Autodesk Inventor part; units mm, degrees
ref_plane "YZ Plane" through (0, 0, 0) normal (1, 0, 0) x (0, 1, 0)
ref_plane "XZ Plane" through (0, 0, 0) normal (0, 1, 0) x (-1, 0, 0)
ref_plane "XY Plane" through (0, 0, 0) normal (0, 0, 1) x (1, 0, 0)
sketch "Sketch1" plane through (0, 0, 0) normal (0, 0, 1) x (1, 0, 0)
  spline S0 degree 3 poles (-30, -5) (-30, -4.3586) (-29.8694, -3.6802) (-29.3471, -2.4395) (-28.9555, -1.8763) (-28.0866, -1.0236) (-27.5672, -0.665) (-27, -0.4174) knots 1.621626 1.621626 1.621626 1.621626 1.814042 1.814042 2.006457 2.006457 2.182648 2.182648 2.182648 2.182648
  line L0 (-25, 0) -> (25, 0)
  spline S1 degree 3 poles (27, -0.4174) (27.5672, -0.665) (28.0866, -1.0236) (28.9555, -1.8763) (29.3471, -2.4395) (29.8694, -3.6802) (30, -4.3586) (30, -5) knots -0.561022 -0.561022 -0.561022 -0.561022 -0.384831 -0.384831 -0.192415 -0.192415 0 0 0 0
  line L1 (30, -5) -> (30, -35)
  spline S2 degree 3 poles (30, -35) (30, -35.6414) (29.8694, -36.3198) (29.3471, -37.5605) (28.9555, -38.1237) (28.0866, -38.9764) (27.5672, -39.335) (27, -39.5826) knots 0 0 0 0 0.192415 0.192415 0.384831 0.384831 0.561022 0.561022 0.561022 0.561022
  line L2 (25, -40) -> (-25, -40)
  line L3 (-30, -35) -> (-30, -5)
  spline S3 degree 3 poles (-27, -39.5826) (-27.5672, -39.335) (-28.0866, -38.9764) (-28.9555, -38.1237) (-29.3471, -37.5605) (-29.8694, -36.3198) (-30, -35.6414) (-30, -35) knots 1.060605 1.060605 1.060605 1.060605 1.236796 1.236796 1.429211 1.429211 1.621626 1.621626 1.621626 1.621626
  arc A0 (-25, 0) -> (-27, -0.4174) centre (-25, -5) ccw
  arc A1 (27, -0.4174) -> (25, 0) centre (25, -5) ccw
  arc A2 (25, -40) -> (27, -39.5826) centre (25, -35) ccw
  arc A3 (-27, -39.5826) -> (-25, -40) centre (-25, -35) ccw
  point P0 (0, 0)
  dimension "d8" = 60
  dimension "d9" = 40
extrude "Extrusion1" add sketch "Sketch1" along normal blind 0.8
sketch "Sketch2" plane through (0, 0, 0) normal (0, 0, -1) x (-1, 0, 0)
  line L0 (-25.5, -10) -> (25.5, -10)
  line L1 (25.5, -10) -> (25.5, -30)
  line L2 (25.5, -30) -> (-25.5, -30)
  line L3 (-25.5, -30) -> (-25.5, -10)
  line L4 (-25.5, -10) -> (25.5, -30) construction
  line L5 (25.5, -10) -> (-25.5, -30) construction
  line L6 (-26.5, -9) -> (26.5, -9)
  line L7 (26.5, -9) -> (26.5, -31)
  line L8 (26.5, -31) -> (-26.5, -31)
  line L9 (-26.5, -31) -> (-26.5, -9)
  line L10 (-26.5, -9) -> (26.5, -31) construction
  line L11 (26.5, -9) -> (-26.5, -31) construction
  point P0 (0, 0)
  point P1 (0, -20)
  point P2 (0, -20)
  dimension "d2" = 51
  dimension "d3" = 20
  dimension "d4" = 53
  dimension "d5" = 22
extrude "Extrusion2" add sketch "Sketch2" along normal blind 2
properties part number "obudowa - budzik v7 plexi" material "Glass"
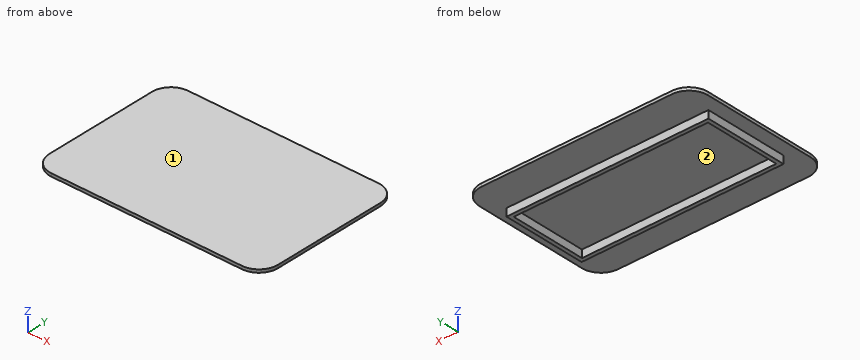
Verification items for the finished model (mm, model axes). Face numbers are marked on the shaded views. Give positions to 0.01 mm unless a question says otherwise; leave off trailing zeros. Order: outer loops, then holes, each group sorted by start corner. A loop starts at its lowest first (then second) coordinate and runs counter-clockwise, first axis right, second up. Notation, with made-up numbers: M -22,-15 L 27,-15 A16 ccw 27,-11 Z; hole C 33,-29.5 d9. An arc over 180 degrees is marked long. Answer as a JSON object with one key per item and string values. Group by question number.
1) Cross-section at A-A (x = -4). Enter the section's corners in (y, z), then the cut area to 3 significant figures.
2) Mould release check, pull along X, two halves, no side actions. Record for the marked faces 1 and 2: released by +X, released by -X, zero draft, split by the parting line, or undercut.
3) Depth check by flat-ended pin: pin 1 Ø1 at (x, z) = (-11, -1) entering from +Y; pin 2 Ø0.6 at (y, z) = (-25, -1) entering from -X; pin 3 Ø16 at (x, y) = (4.5, -21.5) entering from -Z. Enter the tip coordinate at first touch or a pass-through.
4) Cross-section at B-B (y = -20). Enter the section's corners in (x, z).
5) Cross-section at C-C (y = -32). Enter the section's corners in (x, z).
6) Scan lines: line 1 along Y through (x, z) = (-9, -1.2); line 2 along X through (y, z) = (-25, -1.6); line 3 along Z through (x, y) = (-11.5, -23). Record each from-to range of solid material in increasing order. Write a range as [from, to].
Result sheet:
{
 "1": {"outline": "M -40,0 L -31,0 L -31,-2 L -30,-2 L -30,0 L -10,0 L -10,-2 L -9,-2 L -9,0 L 0,0 L 0,0.8 L -40,0.8 Z", "area": "36.0 mm2"},
 "2": {"face 1": "zero draft", "face 2": "undercut"},
 "3": {"pin 1": "stops at y = -9", "pin 2": "stops at x = -26.5", "pin 3": "stops at z = 0"},
 "4": {"outline": "M -30,0 L -26.5,0 L -26.5,-2 L -25.5,-2 L -25.5,0 L 25.5,0 L 25.5,-2 L 26.5,-2 L 26.5,0 L 30,0 L 30,0.8 L -30,0.8 Z"},
 "5": {"outline": "M -30,0 L 30,0 L 30,0.8 L -30,0.8 Z"},
 "6": {"line 1": "y = [-31, -30], [-10, -9]", "line 2": "x = [-26.5, -25.5], [25.5, 26.5]", "line 3": "z = [0, 0.8]"}
}
